```python
from build123d import *

# Parameters (mm, degrees)
PCB_1_2_START = 16.8
SKETCH_1_W    = 32.3
SKETCH_1_H    = 32.3
PCB_1_2_DEPTH = 1.2
PCB_START     = 16.8
SKETCH_2_R    = 1.1
PCB_DEPTH     = 1.2


with BuildPart() as part:
    # 草图1 → PCB装配包络_厚1.2 (new body)
    with BuildSketch(Plane.XY.offset(PCB_1_2_START)):
        Rectangle(SKETCH_1_W, SKETCH_1_H)
    extrude(amount=PCB_1_2_DEPTH)

    # 草图2 → 原厂PCB孔径_非打印放孔 (cut)
    with BuildSketch(Plane.XY.offset(PCB_START)):
        with Locations((-14, -14)):
            Circle(SKETCH_2_R)
        with Locations((-14, 14)):
            Circle(SKETCH_2_R)
        with Locations((14, -14)):
            Circle(SKETCH_2_R)
        with Locations((14, 14)):
            Circle(SKETCH_2_R)
    extrude(amount=PCB_DEPTH, mode=Mode.SUBTRACT)


solid = part.part
```
Model file for the job. Use its own axes, mm. Coordinates: 2 decimals unless noted, no trailing zeros. Order: outer loops, then holes, each group sorted by start corner. A loop starts at its lowest first (then second) coordinate and runs counter-clockwise, first axis right, second up. Notation, with made-up numbers: (-38.75, -1.5) -> (13.25, -1.5) arc R33 cw to (13.25, 29.5) -> close; hole circle Ø4 at (40.25, 40). An arc over 180 degrees is marked (long way). Answer as a JSON object with one key per item and string values. Group by question number.
1) Drill centre lines: L1, parallel to Y at x = -14, z = 17.5; L2, parallel to X at y = 13.5, z = 17.4. Where is each one in solid material? Low to high.
2) Pull direction Y, two halves, no side cores. Call faces 1 (the face through (0, 0, 16.8)), 2 (the face through (0, -16.15, 17)), 3 (the face through (13.762, -15.074, 17.392)): +Y half, -Y half, draft (parallel to the pull), parting line (faces both ways), or undercut.
3) Cut at A-A, the plane y = 14. Write the cut outline in (x, z).
Check values:
{
 "1": {"L1": "y = -16.15 to -15.1, -12.9 to 12.9, 15.1 to 16.15", "L2": "x = -16.15 to -14.98, -13.02 to 13.02, 14.98 to 16.15"},
 "2": {"face 1": "draft", "face 2": "-Y half", "face 3": "undercut"},
 "3": {"outline": "(-16.15, 16.8) -> (-15.1, 16.8) -> (-15.1, 18) -> (-16.15, 18) -> close; (-12.9, 16.8) -> (12.9, 16.8) -> (12.9, 18) -> (-12.9, 18) -> close; (15.1, 16.8) -> (16.15, 16.8) -> (16.15, 18) -> (15.1, 18) -> close"}
}
